Can you work these out from the model? Positions are in its coordinate system, mm. A direction names the side the tool comes from. Round coordinates to 2 decimals unless told otherwise and drop trailing zeros. Write each loop counter-clockwise with the first axis right and the second up, starting at its lowest first coordinate (ties: lowest second). Pieces come first, ordered by that corner, then holes.
Q1. If we section it at C-C (x = -44): Please give me the cut outline in (y, z).
Q2. Please list where these lines run through material, in increasing order: line 1 along Z through (x, y) = (43.5, 43); line 2 along Z through (x, y) = (47.5, 44) (3 decimals); line 3 along Z through (x, y) = (48, 45).
Q3. If we section it at A-A (z = -24.5): Please give me the cut outline in (x, y), plus the area to 3 significant figures.
Q4. We'd pull the mould along Y, two halves only. Please class faces 1 (the flat face through (-25, 19, -71.49)), 2 (the flat face through (46, 49.4, -79)), 3 (the cylindrical face through (45.639, 38.937, -71.312)): +Y half, -Y half, draft (parallel to the pull), parting line (faces both ways), or undercut.
Q5. If we section it at D-D (z = -57.5): Please give me the cut outline in (x, y).
Q6. I'm going to push flat-ended pins straight in: pin 1 Ø1 at (y, z) = (36.5, -130.5) entering from -X; pin 2 Ø1.7 at (x, y) = (43.5, 48) entering from +Z; pin 3 Ø9 at (x, y) = (27.5, 30) entering from -Z; pin 4 Ø3 at (y, z) = (45.4, -95.11) entering from -X. Where does each tip first touch, or does it pass through?
Q7. If we section it at B-B (y = 42): Please give me the cut outline in (x, z), plus the area to 3 significant figures.
Q8. For faces 4 (the flat face through (55, 35.588, -50)), 5 (the flat face through (31.043, 40, -25)), 6 (the flat face through (20.849, 40, -137)), 7 (the flat face through (55, 40, -103.173)), 8 (the flat face through (23, 19, -125.225)), which set-ups out of +Z, -Z, +X, -X, +Y, -Y let a thin tool reach every point of the face, with its end or its side?
Autodesk Inventor part; units mm, degrees
ref_plane "YZ Plane" through (0, 0, 0) normal (1, 0, 0) x (0, 1, 0)
ref_plane "XZ Plane" through (0, 0, 0) normal (0, 1, 0) x (-1, 0, 0)
ref_plane "XY Plane" through (0, 0, 0) normal (0, 0, 1) x (1, 0, 0)
ref_plane "Work Plane1" through (0, 12.7, 0) normal (0, 1, 0) x (1, 0, 0)
sketch "Sketch3" plane through (0, 12.7, 0) normal (0, 1, 0) x (1, 0, 0)
  line L0 (19.05, 32.9956) -> (-3.175, 71.4904)
  line L1 (19.05, 32.9956) -> (27.8488, 32.9956)
  line L2 (-47.625, 71.4904) -> (-52.0244, 79.1104)
  line L3 (27.8488, 32.9956) -> (27.8488, 32.9956)
  line L4 (27.8488, 32.9956) -> (27.8488, 32.9956)
  line L5 (1.2244, 79.1104) -> (-3.175, 71.4904)
  line L6 (-3.175, 71.4904) -> (-47.625, 71.4904)
  line L7 (1.2244, 79.1104) -> (27.8488, 32.9956)
  line L8 (27.8488, 32.9956) -> (19.05, 32.9956)
  line L9 (27.8488, 32.9956) -> (27.8488, 32.9956)
  line L10 (27.8488, 32.9956) -> (27.8488, 32.9956)
  line L11 (1.2244, 79.1104) -> (-52.0244, 79.1104)
  line L12 (19.05, 125.2252) -> (-3.175, 86.7304)
  line L13 (19.05, 125.2252) -> (27.8488, 125.2252)
  line L14 (-47.625, 86.7304) -> (-52.0244, 79.1104)
  line L15 (27.8488, 125.2252) -> (27.8488, 125.2252)
  line L16 (27.8488, 125.2252) -> (27.8488, 125.2252)
  line L17 (1.2244, 79.1104) -> (-3.175, 86.7304)
  line L18 (-3.175, 86.7304) -> (-47.625, 86.7304)
  line L19 (1.2244, 79.1104) -> (27.8488, 125.2252)
  line L20 (27.8488, 125.2252) -> (19.05, 125.2252)
  line L21 (27.8488, 125.2252) -> (27.8488, 125.2252)
  line L22 (27.8488, 125.2252) -> (27.8488, 125.2252)
  line L23 (27.8488, 32.9956) -> (27.8488, 125.2252)
  point P0 (-38.1, 71.4904)
  dimension "d53" = 8.7988
  dimension "d54" = 8.7988
  dimension "d59" = 90
  dimension "d60" = 120
  dimension "d62" = 120
  dimension "d163" = 44.45
  dimension "d173" = 60
ref_plane "Work Plane2" through (0, 88.9, 0) normal (0, 1, 0) x (1, 0, 0)
extrude "Extrusion11" add sketch "Sketch3" along normal blind 12.7 contours L0 L5 L7 L1 | L6 L2 L11 L5
extrude "Extrusion21" add sketch "Sketch3" along normal blind 12.7 contours L11 L14 L18 L17 | L17 L12 L13 L19
extrude "Extrusion22" add sketch "Sketch3" along normal blind 12.7 contours L7 L19 L23
sketch "Sketch15" plane through (27.8488, 12.7, -32.9956) normal (1, 0, 0) x (0, 0, -1)
  line L0 (0, 0) -> (0, 12.7)
  line L1 (0, 12.7) -> (12.0516, 12.7)
  line L2 (0, 12.7) -> (92.2297, 12.7)
  line L3 (92.2297, 0) -> (92.2297, 12.7)
  line L4 (92.2297, 12.7) -> (80.1781, 12.7)
  line L5 (12.0516, 12.7) -> (12.0516, 0)
  line L6 (38.4948, 0) -> (0, 0)
  line L7 (80.1781, 12.7) -> (80.1781, 0)
  line L8 (80.1781, 0) -> (12.0516, 0)
  line L9 (12.0516, 12.7) -> (80.1781, 12.7)
  point P0 (-32.9956, -12.7)
  point P1 (38.4948, 0)
  dimension "d180" = 12.0516
  dimension "d181" = 12.0516
extrude "Extrusion23" add sketch "Sketch15" along normal blind 22.86 contours L5 L2 L7 L8 L6
sketch "Sketch16" plane through (0, 25.4, 0) normal (0, 1, 0) x (1, 0, 0)
  line L0 (27.8488, 45.0472) -> (50.7088, 45.0472)
  line L1 (50.7088, 45.0472) -> (50.7088, 55.0472)
  line L2 (50.7088, 113.1736) -> (50.7088, 45.0472)
  line L3 (27.8488, 32.9956) -> (27.8488, 45.0472)
  line L4 (27.8488, 45.0472) -> (27.8488, 55.0472)
  line L5 (27.8488, 55.0472) -> (50.7088, 55.0472)
  line L6 (27.8488, 45.0472) -> (17.8488, 45.0472)
  line L7 (17.8488, 45.0472) -> (17.8488, 55.0472)
  line L8 (17.8488, 55.0472) -> (27.8488, 55.0472)
  point P0 (0, 0)
  dimension "d184" = 10
  dimension "d185" = 10
  dimension "d199" = 10
  dimension "d200" = 10
extrude "Extrusion24" add sketch "Sketch16" along normal blind 18.288
sketch "Sketch18" plane through (27.8488, 12.7, -45.0472) normal (0, 0, 1) x (1, 0, 0)
  line L0 (-7, 22.988) -> (-7, 30.988)
  line L1 (-7, 30.988) -> (-7, 22.988)
  line L2 (-7, 22.988) -> (3.1943, 22.988)
  line L3 (3.1943, 22.988) -> (3.1943, 30.988)
  line L4 (3.1943, 30.988) -> (-7, 30.988)
  point P0 (-27.8488, -12.7)
extrude "Extrusion26" add sketch "Sketch18" along normal blind 48
sketch "Sketch19" plane through (50.7088, 12.7, -32.9956) normal (1, 0, 0) x (0, 0, -1)
  line L0 (12.0516, 30.988) -> (22.0516, 30.988)
  line L1 (12.0516, 22.988) -> (22.0516, 22.988)
  line L2 (12.0516, 30.988) -> (12.0516, 22.988)
  line L3 (12.0516, 22.988) -> (22.0516, 22.988)
  line L4 (22.0516, 22.988) -> (22.0516, 30.988)
  line L5 (22.0516, 30.988) -> (12.0516, 30.988)
  point P0 (-32.9956, -12.7)
extrude "Extrusion27" add sketch "Sketch19" along normal blind 8
sketch "Sketch20" plane through (27.8488, 12.7, -45.0472) normal (0, 0, 1) x (1, 0, 0)
  line L0 (-10, 30.988) -> (30.86, 30.988)
  line L1 (30.86, 30.988) -> (23.2839, 30.988)
  line L2 (30.86, 30.988) -> (30.86, 22.988)
  line L3 (30.86, 30.988) -> (30.86, 22.988)
  line L4 (23.2839, 30.988) -> (23.2839, 22.988)
  line L5 (22.86, 22.988) -> (30.86, 22.988)
  line L6 (23.2839, 22.988) -> (30.86, 22.988)
  point P0 (-27.8488, -12.7)
  point P1 (-7, 30.988)
extrude "Extrusion28" add sketch "Sketch20" along normal blind 48
sketch "Sketch21" plane through (31.0431, 35.688, -45.0472) normal (1, 0, 0) x (0, 0, -1)
  line L0 (0, 8) -> (-48, 8)
  line L1 (-48, 8) -> (-40.0559, 8)
  line L2 (0, 0) -> (-48, 0)
  line L3 (-48, 8) -> (-40.0559, 8)
  line L4 (-40.0559, 8) -> (-40.0559, 0)
  line L5 (-40.0559, 0) -> (-48, 0)
  line L6 (-48, 0) -> (-48, 8)
  point P0 (-45.0472, -35.688)
  point P1 (-40.0559, 8)
extrude "Extrusion29" add sketch "Sketch21" along normal blind 24
sketch "Sketch22" plane through (20.8488, 35.688, -45.0472) normal (0, -1, 0) x (1, 0, 0)
  line L0 (29.86, -10) -> (29.86, 0)
  line L1 (29.86, 0) -> (29.86, -10)
  line L2 (-3, -10) -> (37.86, -10)
  line L3 (29.86, -10) -> (37.86, -10)
  line L4 (37.86, -10) -> (37.86, 0)
  line L5 (37.86, -10) -> (37.86, 48)
  line L6 (37.86, 0) -> (29.86, 0)
  line L7 (10.1943, 0) -> (30.2839, 0)
  point P0 (-20.8488, 45.0472)
extrude "Extrusion30" add sketch "Sketch22" along normal blind 0.1
sketch "Sketch23" plane through (27.8488, 12.7, -125.2252) normal (1, 0, 0) x (0, 0, -1)
  line L0 (0, 12.7) -> (-38.4948, 12.7)
  line L1 (0, 12.7) -> (-92.23, 12.7)
  line L2 (-92.23, 12.7) -> (-46.115, 12.7)
  line L3 (-46.115, 12.7) -> (-46.115, -5.4256)
  point P0 (-125.2252, -12.7)
  dimension "d206" = 92.23
  dimension "d207" = 46.115
ref_plane "Work Plane5" through (27.8488, 25.4, -79.1102) normal (0, 0, 1) x (0, -1, 0)
mirror "Mirror2" about plane through (27.8488, 25.4, -79.1102) normal (0, 0, 1) of "Extrusion24", "Extrusion26", "Extrusion27", "Extrusion28", "Extrusion29", "Extrusion30"
sketch "Sketch24" plane through (0, 25.4, 0) normal (0, 1, 0) x (1, 0, 0)
  line L0 (50.7088, 103.1733) -> (50.7088, 55.0472)
  line L1 (50.7088, 55.0472) -> (50.7088, 103.1733)
  line L2 (50.7088, 103.1733) -> (40.7088, 103.1733)
  line L3 (58.7088, 103.1733) -> (17.8488, 103.1733)
  line L4 (40.7088, 103.1733) -> (40.7088, 55.0472)
  line L5 (17.8488, 55.0472) -> (50.7088, 55.0472)
  line L6 (40.7088, 55.0472) -> (50.7088, 55.0472)
  point P0 (0, 0)
  dimension "d209" = 10
  dimension "d210" = 90
extrude "Extrusion31" add sketch "Sketch24" along normal blind 24
sketch "Sketch25" plane through (40.7088, 25.4, -103.1733) normal (-1, 0, 0) x (0, 0, 1)
  line L0 (0, 18.288) -> (0, 24)
  line L1 (48.1261, 0) -> (0, 0)
  line L2 (0, 24) -> (48.1261, 24)
  line L3 (48.1261, 24) -> (48.1261, 0)
  line L4 (48.1261, 0) -> (0, 0)
  line L5 (0, 0) -> (0, 24)
  line L6 (0, 24) -> (24.0631, 24)
  line L7 (24.0631, 24) -> (24.0631, 12)
  circle A0 centre (24.0631, 12) radius 1.55
  line L8 (24.0631, 12) -> (24.0631, 20)
  circle A1 centre (24.0631, 20) radius 1.55
  line L9 (24.0631, 12) -> (24.0631, 4)
  circle A2 centre (24.0631, 4) radius 1.55
  line L10 (24.0631, 12) -> (16.0631, 12)
  line L11 (16.0631, 12) -> (32.0631, 12)
  circle A3 centre (16.0631, 12) radius 1.55
  circle A4 centre (32.0631, 12) radius 1.55
  circle A5 centre (0.0631, 12) radius 1.55
  circle A6 centre (8.0631, 12) radius 1.55
  circle A7 centre (8.0631, 20) radius 1.55
  circle A8 centre (16.0631, 12) radius 1.55
  circle A9 centre (8.0631, 4) radius 1.55
  circle A10 centre (32.0631, 12) radius 1.55
  circle A11 centre (40.0631, 12) radius 1.55
  circle A12 centre (40.0631, 20) radius 1.55
  circle A13 centre (48.0631, 12) radius 1.55
  circle A14 centre (40.0631, 4) radius 1.55
  circle A15 centre (16.0631, 12) radius 1.55
  circle A16 centre (24.0631, 12) radius 1.55
  circle A17 centre (24.0631, 20) radius 1.55
  circle A18 centre (32.0631, 12) radius 1.55
  circle A19 centre (24.0631, 4) radius 1.55
  point P0 (103.1733, -25.4)
  dimension "d216" = 3.1
  dimension "d217" = 8
  dimension "d218" = 3.1
  dimension "d219" = 8
  dimension "d220" = 3.1
  dimension "d221" = 8
  dimension "d222" = 16
  dimension "d223" = 3.1
  dimension "d224" = 3.1
  dimension "d229" = 16
  dimension "d232" = 16
extrude "Extrusion32" cut sketch "Sketch25" against normal blind 14.75 contours A4 | A2 | A3 | A0 L11 L7 | L7 L10 A0 | A1 L7 | L7 A1 | L11 A0 L9 | L9 A0 L10 | A6 | A7 | A9 | A11 | A12 | A14
properties part number "HorizontalGrabberMain"
A:
1. outline: (12.7, -86.73) - (25.4, -86.73) - (25.4, -71.49) - (12.7, -71.49) - close
2. line 1: z = -161.17 to -153.23, -113.17 to -45.05, -4.99 to 2.95
2. line 2: z = -103.173 to -95.775, -94.445 to -79.775, -78.445 to -63.775, -62.445 to -55.047
2. line 3: z = -103.17 to -96.61, -93.61 to -80.61, -77.61 to -64.61, -61.61 to -55.05
3. outline: (20.85, 35.69) - (31.04, 35.69) - (31.04, 43.69) - (20.85, 43.69) - close; (51.13, 35.69) - (58.71, 35.69) - (58.71, 43.69) - (51.13, 43.69) - close
3. area: 142 mm2
4. face 1: draft
4. face 2: +Y half
4. face 3: undercut
5. outline: (4.9, 12.7) - (50.71, 12.7) - (50.71, 49.4) - (40.71, 49.4) - (40.71, 25.4) - (4.9, 25.4) - close
6. pin 1: stops at x = 20.85
6. pin 2: stops at z = -55.05
6. pin 3: stops at z = -113.17
6. pin 4: passes through
7. outline: (17.85, -113.17) - (20.85, -113.17) - (20.85, -161.17) - (58.71, -161.17) - (58.71, -103.17) - (50.71, -103.17) - (50.71, -55.05) - (58.71, -55.05) - (58.71, 2.95) - (20.85, 2.95) - (20.85, -45.05) - (17.85, -45.05) - (17.85, -55.05) - (40.71, -55.05) - (40.71, -103.17) - (17.85, -103.17) - close; hole (31.04, -153.23) - (51.13, -153.23) - (51.13, -113.17) - (31.04, -113.17) - close; hole (31.04, -45.05) - (51.13, -45.05) - (51.13, -4.99) - (31.04, -4.99) - close
7. area: 3,320 mm2
8. face 4: +Z, -Z, +X, -Y
8. face 5: +Y, -Y
8. face 6: -Z, -X, +Y
8. face 7: +X, +Y, -Y
8. face 8: -Z, +X, -X, -Y
